Verification items for the finished model (mm, model axes). A direction names the side the tool comes from. Round coordinates to 2 decimals unless told otherwise and drop trailing zeros. Write each loop counter-clockwise with the first axis right and the second up, starting at its lowest first coordinate (ties: lowest second). Pieces come first, ordered by that corner, then holes. Notation, with made-up numbers: (13, -24) - (48, -24) arc R15 cw to (48, -2) - close; hole circle Ø7 at (13, 56). An arc over 180 degrees is marked (long way). Answer as a JSON object with one key per item and string values.
Solid Edge part; units mm, degrees
sketch "Sketch1" plane through (0, 0, 0) normal (0, 0, 1) x (1, 0, 0)
  line L0 (0, 0) -> (0, 2.35)
  line L1 (0, 2.35) -> (0.325, 2.35)
  line L2 (0.325, 2.35) -> (1.3873, 1.2877)
  arc A0 (1.3873, 1.2877) -> (1.8115, 1.112) centre (1.8115, 1.712) ccw
  line L3 (1.8115, 1.112) -> (2.161, 1.112)
  line L4 (2.161, 1.112) -> (2.4, 1.25)
  line L5 (2.4, 1.25) -> (20, 1.25)
  line L6 (20, 1.25) -> (20, 0)
  line L7 (20, 0) -> (0, 0)
revolve "RevolvedProtrusion1" add sketch "Sketch1" angle 360 about axis through (20, 0, 0) along (-1, 0, 0)
sketch "Sketch2" plane through (0, 0, 0) normal (0, 0, 1) x (1, 0, 0)
  line L0 (-1, 1.45) -> (-1, -1.45)
  line L1 (-1, -1.45) -> (0.75, -1.45)
  line L2 (0.75, -1.45) -> (2.1855, -0.3625)
  line L3 (2.1855, -0.3625) -> (2.1855, 0.3625)
  line L4 (2.1855, 0.3625) -> (0.75, 1.45)
  line L5 (0.75, 1.45) -> (-1, 1.45)
extrude "ExtrudedCutout_1" cut sketch "Sketch2" against normal blind 0.3625 and the other way blind 0.3625
sketch "Sketch3" plane through (0, 0, 0) normal (0, -1, 0) x (1, 0, 0)
  line L0 (-1, -1.45) -> (-1, 1.45)
  line L1 (-1, 1.45) -> (0.75, 1.45)
  line L2 (0.75, 1.45) -> (2.2, 0.3625)
  line L3 (2.2, 0.3625) -> (2.2, -0.3625)
  line L4 (2.2, -0.3625) -> (0.75, -1.45)
  line L5 (0.75, -1.45) -> (-1, -1.45)
extrude "ExtrudedCutout_2" cut sketch "Sketch3" against normal blind 0.358 and the other way blind 0.358
properties part number "SFS FN 406 283597 Senkschraube ISO 7046-1 Stahl 4.8 verzinkt blau M2.5x20-H"
1. Mould release check, pull along X, two halves, no side actions. Record for faces 1 (the face through (1.465, -0.005, 0.914)), 2 (the face through (1, -0.358, 1)), 3 (the face through (1.99, 1.06, 0.33)): released by +X, released by -X, zero draft, split by the parting line, or undercut.
Completed:
{"face 1": "released by -X", "face 2": "zero draft", "face 3": "undercut"}
2. Access from +Z, -Z, +X, -X, +Y, -Y to the whole of each face (thin tool, end or side, straight path). Record for faces 4 (the face through (1, 1, 0.362)), 5 (the face through (11.32, -0.27, -1.22)), 6 (the face through (0, -1, -1)).
Completed:
{"face 4": "-X", "face 5": "+X", "face 6": "+Z, -Z, -X, +Y, -Y"}
3. Material ranges on probe 1 along Y at (x, z) = (12.75, -0.05); probe 2 along Y at (x, z) = (1.25, 0.55); probe 3 along X at (y, z) = (-1.95, 0.95), recorded low to high. Write a range as from..to.
Completed:
{"probe 1": "y = -1.25..1.25", "probe 2": "y = -1.31..-0.36, 0.36..1.31", "probe 3": "x = 0..0.51"}
4. Cross-section at C-C (x = 11.25). Record the boundary of the cut face in (y, z).
Completed:
{"outline": "circle Ø2.5 at (0, 0)"}
5. Go/stop test with flat-tipped pins: pin 1 (0.9 mm diameter, centred on x = 1.5, y = -1, fed in from +Z); pin 2 (2 mm diameter, centred on x = 4.5, z = 1.5, fed in from -Y); pin 3 (0.5 mm diameter, centred on x = 1, y = 1, fed in from +Z). Record where each tip stops, or that it passes through.
Completed:
{"pin 1": "stops at z = 1.36", "pin 2": "stops at y = -1.15", "pin 3": "stops at z = 1.68"}
